Input: dimensioned drawing with shaded views. Units: mm. Origin: part minimum x, y, z. A direction names the side the tool comes from. Round coordinates to 2 decimals unless told otherwise and drop trailing zeros. Order: outer loops, then holes, each group sorted by start corner. A loop starts at its lowest first (then second) coordinate and runs counter-clockwise, first axis right, second up. Notation, with made-up numbers: (5, 79) - (18, 79) arc R28 ccw to (18, 97) - close; hole circle Ø4 at (75, 33.5). An arc over 180 degrees is marked (long way). Put each result on its own line as item: value. Start each with the question number.
(1) Material intervals for L1, parallel to Z at x = 36, y = 93; L2, parallel to X at y = 29.5, z = 49, sorted ascending. Write a range as [from, to].
(2) Access query for the marked faces 1 and 2. Directions: +Z, -Z, +X, -X, +Y, -Y. A direction counts if a zero-diameter tool reaches every point of the face in a straight line with its end or side. Return the directions, or none.
(3) Section B-B (y = 86). Output: boundary loops of the cut face in (x, z).
(4) Section A-A (z = 54.5). Output: boundary loops of the cut face in (x, y).
(5) Section C-C (x = 46). Output: boundary loops of the cut face in (y, z).
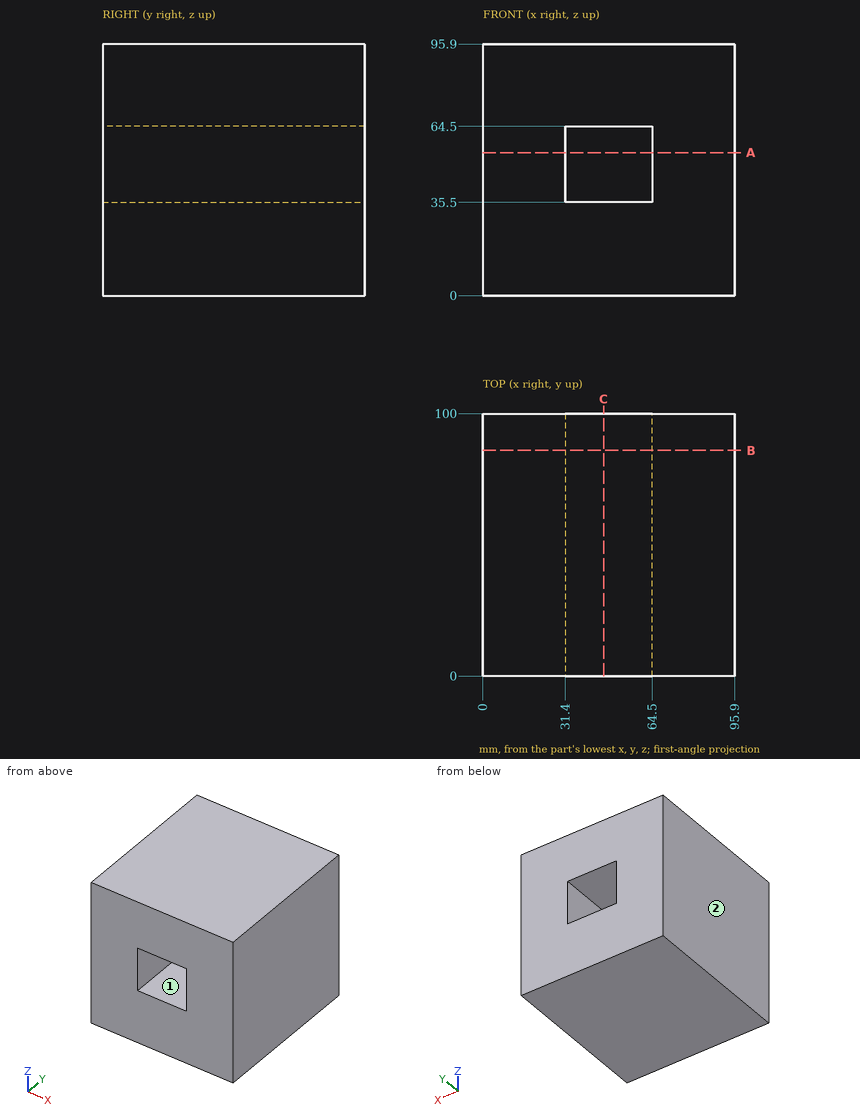
Checks:
1. L1: z = [0, 35.5], [64.5, 95.9]
1. L2: x = [0, 31.4], [64.5, 95.9]
2. face 1: +Y, -Y
2. face 2: +Z, -Z, -X, +Y, -Y
3. outline: (0, 0) - (95.9, 0) - (95.9, 95.9) - (0, 95.9) - close; hole (31.4, 35.5) - (64.5, 35.5) - (64.5, 64.5) - (31.4, 64.5) - close
4. outline: (0, 0) - (31.4, 0) - (31.4, 100) - (0, 100) - close; (64.5, 0) - (95.9, 0) - (95.9, 100) - (64.5, 100) - close
5. outline: (0, 0) - (100, 0) - (100, 35.5) - (0, 35.5) - close; (0, 64.5) - (100, 64.5) - (100, 95.9) - (0, 95.9) - close
